```python
from build123d import *

# Parameters (mm, degrees)
PAD_DEPTH       = 22
POCKET_DEPTH    = 20
SKETCH002_W     = 12
SKETCH002_H     = 12
POCKET001_DEPTH = 7
SKETCH003_R     = 2
POCKET002_DEPTH = 15.001
SKETCH004_R     = 1.75
POCKET003_DEPTH = 6
SKETCH005_R     = 1.75
POCKET004_DEPTH = 6
POCKET005_DEPTH = 4
POCKET006_DEPTH = 4
POCKET007_DEPTH = 0.2


with BuildPart() as part:
    # Sketch → Pad (new body)
    with BuildSketch(Plane.XY):
        Polygon((-32.5, -39), (-32.5, -24.5), (-21, -24.5), (-21, -3.5), (-25, -3.5), (-25, 3.5), (-21, 3.5), (-21, 24.5), (-32.5, 24.5), (-32.5, 39), (32.5, 39), (32.5, 24.5), (21, 24.5), (21, 13.5), (31, 13.5), (31, 3.5), (25, 3.5), (25, -3.5), (31, -3.5), (31, -13.5), (21, -13.5), (21, -24.5), (32.5, -24.5), (32.5, -39), align=None)
    extrude(amount=PAD_DEPTH)

    # Sketch001 → Pocket (cut)
    with BuildSketch(Plane.XY.offset(22)):
        Polygon((-29, 39), (-29, 30), (-21, 30), (-21, 1), (21, 1), (21, 30), (29, 30), (29, 39), align=None)
        Polygon((21, -1), (-21, -1), (-21, -30), (-29, -30), (-29, -39), (29, -39), (29, -30), (21, -30), align=None)
    extrude(amount=-POCKET_DEPTH, mode=Mode.SUBTRACT)

    # Sketch002 → Pocket001 (cut)
    with BuildSketch(Plane.XY.offset(22)):
        with Locations((27, 9.25)):
            Rectangle(SKETCH002_W, SKETCH002_H)
        with Locations((27, -9.25)):
            Rectangle(SKETCH002_W, SKETCH002_H)
    extrude(amount=-POCKET001_DEPTH, mode=Mode.SUBTRACT)

    # Sketch003 → Pocket002 (cut, through all)
    with BuildSketch(Plane.XY.offset(15)):
        with Locations((26, 8.5)):
            Circle(SKETCH003_R)
        with Locations((26, -8.5)):
            Circle(SKETCH003_R)
    extrude(amount=-POCKET002_DEPTH, mode=Mode.SUBTRACT)

    # Sketch004 → Pocket003 (cut)
    with BuildSketch(Plane.XZ.offset(30)):
        with Locations((-25.5, 17.5)):
            Circle(SKETCH004_R)
        with Locations((-25.5, 7.5)):
            Circle(SKETCH004_R)
        with Locations((25.5, 17.5)):
            Circle(SKETCH004_R)
        with Locations((25.5, 7.5)):
            Circle(SKETCH004_R)
    extrude(amount=-POCKET003_DEPTH, mode=Mode.SUBTRACT)

    # Sketch005 → Pocket004 (cut)
    with BuildSketch(Plane(origin=(0, 30, 0), x_dir=(-1, 0, 0), z_dir=(0, 1, 0))):
        with Locations((-25.5, 17.5)):
            Circle(SKETCH005_R)
        with Locations((-25.5, 7.5)):
            Circle(SKETCH005_R)
        with Locations((25.5, 17.5)):
            Circle(SKETCH005_R)
        with Locations((25.5, 7.5)):
            Circle(SKETCH005_R)
    extrude(amount=-POCKET004_DEPTH, mode=Mode.SUBTRACT)

    # Sketch007 → Pocket005 (cut)
    with BuildSketch(Plane.XZ.offset(-24.5)):
        Polygon((-25.5, 21.021837), (-28.55, 19.260918), (-28.55, 15.739082), (-25.5, 13.978163), (-22.45, 15.739082), (-22.45, 19.260918), align=None)
        Polygon((-25.5, 11.021837), (-28.55, 9.260918), (-28.55, 5.739082), (-25.5, 3.978163), (-22.45, 5.739082), (-22.45, 9.260918), align=None)
    pocket005 = extrude(amount=-POCKET005_DEPTH, mode=Mode.SUBTRACT)

    # Mirrored: Pocket005 across Sketch007 V_Axis
    add(pocket005.mirror(Plane(origin=(0, 24.5, 0), x_dir=(0, -1, 0), z_dir=(1, 0, 0))), mode=Mode.SUBTRACT)

    # Sketch006 → Pocket006 (cut)
    with BuildSketch(Plane(origin=(0, -24.5, 0), x_dir=(-1, 0, 0), z_dir=(0, 1, 0))):
        Polygon((-25.5, 21.021837), (-28.55, 19.260918), (-28.55, 15.739082), (-25.5, 13.978163), (-22.45, 15.739082), (-22.45, 19.260918), align=None)
        Polygon((-25.5, 11.021837), (-28.55, 9.260918), (-28.55, 5.739082), (-25.5, 3.978163), (-22.45, 5.739082), (-22.45, 9.260918), align=None)
    pocket006 = extrude(amount=-POCKET006_DEPTH, mode=Mode.SUBTRACT)

    # Mirrored001: Pocket006 across Sketch006 V_Axis
    add(pocket006.mirror(Plane(origin=(0, -24.5, 0), x_dir=(0, 1, 0), z_dir=(-1, 0, 0))), mode=Mode.SUBTRACT)

    # Sketch008 → Pocket007 (cut)
    with BuildSketch(Plane.XY.offset(2)):
        Polygon((9.5, 13.5), (-9.5, 13.5), (-9.5, 27), (-14, 27), (-14, 28.5), (-9.5, 28.5), (-9.5, 31.5), (-6, 31.5), (-6, 34), (-3.7, 34), (-3.7, 31.5), (6.5, 31.5), (9.5, 28.5), (14, 28.5), (14, 27), (9.5, 27), align=None)
    pocket007 = extrude(amount=-POCKET007_DEPTH, mode=Mode.SUBTRACT)

    # Mirrored002: Pocket007 across Sketch008 H_Axis
    add(pocket007.mirror(Plane(origin=(0, 0, 2), x_dir=(0, 0, 1), z_dir=(0, 1, 0))), mode=Mode.SUBTRACT)


solid = part.part
```
Model file for the job. Use its own axes, mm. A direction names the side the tool comes from. Round coordinates to 2 decimals unless told otherwise and drop trailing zeros. Write each loop counter-clockwise with the first axis right and the second up, starting at its lowest first coordinate (ties: lowest second). Pieces come first, ordered by that corner, then holes. Notation, with made-up numbers: (68.5, 44.5) -> (105.5, 44.5) arc R33 cw to (105.5, 75.5) -> close; hole circle Ø8 at (83.5, -8). An arc over 180 degrees is marked (long way). Answer as CSV lines item,"result".
1. Slice it at C-C, the plane y = -17.5. List the corners of the cut face in (x, z), plus the area to 3 significant figures.
Resolved:
outline,"(-21, 0) -> (21, 0) -> (21, 2) -> (9.5, 2) -> (9.5, 1.8) -> (-9.5, 1.8) -> (-9.5, 2) -> (-21, 2) -> close"
area,"80.2 mm²"
2. Tool access for faces 4 (the face through (27, 24.5, 11)), 5 (the face through (-27.046, 26.472, 14.871)), 6 (the face through (-26.79, -29.26, 18.68)), 7 (the face through (-25, 0, 11)), 8 (the face through (23, 3.25, 19)): list every direction of +Z, -Z, +X, -X, +Y, -Y with a clear straight run to the whole face (end or side of a thin tool).
Resolved:
face 4,"+Z, -Z, +X"
face 5,"none"
face 6,"-Y"
face 7,"+Z, -Z, -X"
face 8,"+Z, +X"
3. Slice it at A-A, the plane y = -8.5. List the corners of the cut face in (x, z).
Resolved:
outline,"(-21, 0) -> (24, 0) -> (24, 15) -> (21, 15) -> (21, 2) -> (-21, 2) -> close; (28, 0) -> (31, 0) -> (31, 15) -> (28, 15) -> close"
4. Pin check, flat tips, straight feed: pin 1 Ø3 at (y, z) = (11.5, 2.5) entering from +X; pin 2 Ø4 at (x, z) = (0.5, 5.5) entering from +Y; pin 3 Ø3 at (x, z) = (24, 10) entering from -Y; pin 4 Ø1 at (x, y) = (18.5, -3) entering from -Z. Stop position of each tip, or through.
Resolved:
pin 1,"x = 31"
pin 2,"y = 1"
pin 3,"y = -30"
pin 4,"z = 0"
5. Mould opens along X. For faces 1 (the face through (27, -24.5, 11)), 2 (the face through (25, 0, 11)), 3 (the face through (-27.004, 26.472, 10.154)) say: +X half, -X half, draft (parallel to the pull), parting line (faces both ways), or undercut.
Resolved:
face 1,"draft"
face 2,"+X half"
face 3,"undercut"
6. Drill centre lines: line 1 (Z direction, x = -25.5, y = -29); line 2 (Y direction, x = 28.5, z = 7.75); line 3 (Y direction, x = 22, z = 6.5). Where is each one in solid material? Low to high.
Resolved:
line 1,"0 to 5.75, 9.25 to 15.75, 19.25 to 22"
line 2,"-30 to -28.5, -13.5 to -3.5, 3.5 to 13.5, 28.5 to 30"
line 3,"-30 to -24.5, -13.5 to 13.5, 24.5 to 30"
7. Slice it at D-D, the plane z = 7.5. State how many separate pieces and enclosed holes the cut face has, plus the area to 3 significant figures.
Resolved:
separate pieces,"9"
enclosed holes,"2"
area,"575 mm²"
8. Slice it at B-B, the plane x = -17. List the corners of the cut face in (y, z), plus the area to 3 significant figures.
Resolved:
outline,"(-39, 0) -> (39, 0) -> (39, 2) -> (1, 2) -> (1, 22) -> (-1, 22) -> (-1, 2) -> (-39, 2) -> close"
area,"196 mm²"
